from build123d import *

# Parameters (mm, degrees)
F0_W     = 374.65
F0_H     = 174.625
F1_DEPTH = 12.7
F2_W     = 350.8375
F2_H     = 6.35
F2_W_2   = 6.35
F2_H_2   = 161.925
F2_W_3   = 17.4625
F3_DEPTH = 6.35
F4_SIZE2 = 5.08
F4_SIZE  = 17.4625
F2_W_4   = 50.8
F2_H_3   = 50.8
F5_DEPTH = 6.35
F6_R     = 25.39999
F7_SIZE2 = 6.34999
F7_SIZE  = 25.39999


# Not quite as in the source:
# - a fillet or chamfer is up to 0.001 mm smaller than in the source, because OpenCascade refuses the exact size


with BuildPart() as f1:
    # F0 (on Front) → F1 (new body)
    with BuildSketch(Plane.XZ):
        Rectangle(F0_W, F0_H)
    extrude(amount=F1_DEPTH)

    # F2 (on face) → F3 (cut)
    with BuildSketch(Plane.XZ.offset(12.7)):
        with Locations((-5.55625, 84.1375)):
            Rectangle(F2_W, F2_H)
        with Locations((-184.15, 84.1375)):
            Rectangle(F2_W_2, F2_H)
        with Locations((-184.15, 0)):
            Rectangle(F2_W_2, F2_H_2)
        with Locations((-184.15, -84.1375)):
            Rectangle(F2_W_2, F2_H)
        with Locations((-5.55625, -84.1375)):
            Rectangle(F2_W, F2_H)
        with Locations((178.59375, -84.1375)):
            Rectangle(F2_W_3, F2_H)
        with Locations((178.59375, 84.1375)):
            Rectangle(F2_W_3, F2_H)
    extrude(amount=-F3_DEPTH, mode=Mode.SUBTRACT)

    # F4
    f4_edges = [f1.edges().sort_by_distance(p)[0] for p in [
        (187.325, -12.7, 0),
    ]]
    f4_side = f1.faces().sort_by_distance((3.175, -12.7, 0))[0]
    chamfer(f4_edges, length=F4_SIZE, length2=F4_SIZE2, reference=f4_side)

    # F2 (on face) → F5 (cut)
    with BuildSketch(Plane.XZ.offset(12.7)):
        with Locations((136.525, 0)):
            Rectangle(F2_W_4, F2_H_3)
    extrude(amount=-F5_DEPTH, mode=Mode.SUBTRACT)

    # F6 (radius 25.4 in the source; OpenCascade refuses exactly that, so slightly less here)
    f6_edges = [f1.edges().sort_by_distance(p)[0] for p in [
        (111.125, -9.525, -25.4),
        (111.125, -9.525, 25.4),
    ]]
    fillet(f6_edges, radius=F6_R)

    # F7 (size 25.4 and 6.35 in the source; OpenCascade refuses exactly that, so slightly less here)
    f7_edges = [f1.edges().sort_by_distance(p)[0] for p in [
        (118.564485, -6.35, -17.960515),
    ]]
    f7_side = f1.faces().sort_by_distance((138.896085, -6.35, 0))[0]
    chamfer(f7_edges, length=F7_SIZE, length2=F7_SIZE2, reference=f7_side)


solid = f1.part
CAD build for the part. Positions are in the model's coordinates, mm. A direction names the side the tool comes from. Give positions to 0.01 mm unless a question says otherwise; leave off trailing zeros. Write each loop counter-clockwise with the first axis right and the second up, starting at its lowest first coordinate (ties: lowest second). Pieces come first, ordered by that corner, then holes. Notation, with made-up numbers: (21.25, 63.5) -> (66.25, 63.5) arc R17 ccw to (66.25, 91.5) -> close; hole circle Ø9 at (62, 82.5). An arc over 180 degrees is marked (long way). Return JSON: item names as keys, results as strings.
Item 1: Drill centre lines: probe 1 along Z at (x, y) = (-116.5, -9); probe 2 along Y at (x, z) = (151.5, -25); probe 3 along Y at (x, z) = (161.5, -17.5) (3 decimals). Where is each one in solid material? Low to high.
Answer below:
{"probe 1": "z = -80.96 to 80.96", "probe 2": "y = -12.6 to 0", "probe 3": "y = -10.725 to 0"}
Item 2: Tool access for faces 4 (the flat face through (161.925, -10, 0)), 5 (the flat face through (-187.325, -3, -1)), 6 (the flat face through (-180.975, -10, -1)), 7 (the flat face through (6, -10, -80.962)): list every direction of +Z, -Z, +X, -X, +Y, -Y with a clear straight run to the whole face (end or side of a thin tool).
Answer below:
{"face 4": "-Y", "face 5": "+Z, -Z, -X, +Y, -Y", "face 6": "+Z, -Z, -X, -Y", "face 7": "-Z, +X, -X, -Y"}
Item 3: Band-saw the part on B-B (x = -95). List the corners of the cut face in (y, z), then the cut area to 3 significant figures.
Answer below:
{"outline": "(-12.7, -80.96) -> (-6.35, -80.96) -> (-6.35, -87.31) -> (0, -87.31) -> (0, 87.31) -> (-6.35, 87.31) -> (-6.35, 80.96) -> (-12.7, 80.96) -> close", "area": "2,140 mm2"}
Item 4: Two-plate mould, pull along Z, no slides. Class faces 1 (the flat face through (149.4, -9.57, -12.88)), 2 (the flat face through (178.716, -10.124, -1.133)), 3 (the flat face through (1, -10, 80.962)): +Z half, -Z half, draft (parallel to the pull), parting line (faces both ways), or undercut.
Answer below:
{"face 1": "undercut", "face 2": "draft", "face 3": "+Z half"}
Item 5: Drop flat-ended pins along their axis: pin 1 (2 mm diameter, centred on x = -145, y = -10.5, fed in from +Z); pin 2 (1.9 mm diameter, centred on y = -9, z = -8, fed in from -X) (3 decimals); pin 3 (1.9 mm diameter, centred on x = -82, y = -9, fed in from -Z). Give the stop position or say it passes through.
Answer below:
{"pin 1": "stops at z = 80.96", "pin 2": "stops at x = -180.975", "pin 3": "stops at z = -80.96"}
